Verification items for the finished model (mm, model axes). Face numbers are marked on the shaded views. A direction names the side the tool comes from. Round coordinates to 2 decimals unless told otherwise and drop trailing zeros. Order: outer loops, then holes, each group sorted by start corner. A loop starts at its lowest first (then second) coordinate and runs counter-clockwise, first axis right, second up. Notation, with made-up numbers: (-4, 18) -> (38, 18) arc R17 ccw to (38, 40) -> close; hole circle Ø5 at (6, 58). An arc over 180 degrees is marked (long way). Return JSON: item names as keys, results as strings. Group by question number.
Item 1: Sectioned sample at A-A on x = 0. Record the cut outline in (y, z).
Item 2: Depth check by flat-ended pin: pin 1 Ø1 at (x, z) = (-5, 0.5) entering from -Y. Enter the tip coordinate at first touch or a pass-through.
Item 3: Sectioned sample at C-C on z = 0.5. Record the cut outline in (x, y) (1 decimal), plus the area to 3 significant figures.
Item 4: Sectioned sample at B-B on y = 0. Record the cut outline in (x, z) (3 decimals), plus the area to 4 significant figures.
Item 5: Access from +Z, -Z, +X, -X, +Y, -Y to the whole of each face (thin tool, end or side, straight path). Record for the marked faces 1 and 2.
Item 6: Scan lines: probe 1 along Y at (x, z) = (4.5, 1); probe 2 along Y at (x, z) = (0.75, 1.05); probe 3 along X at (y, z) = (1, 0.35) (3 decimals). Record each from-to range of solid material in increasing order. Write a range as from..to.
Item 7: Sectioned sample at D-D on y = 38. Record the cut outline in (x, z).
Item 8: Draft check along Y on the marked faces 3, 4 and 5. Enter one of: pulls with the +Y half, pulls with the -Y half, needs draft (parallel to the pull), parting line crosses it, or undercut.
```python
from build123d import *

# Parameters (mm, degrees)
F0_R     = 5.4
F1_DEPTH = 1.5
F3_DEPTH = 1.5
F6_DEPTH = 1.5
F7_R     = 1


with BuildPart() as f1:
    # F0 (on Top) → F1 (new body, symmetric)
    with BuildSketch(Plane.XY):
        Circle(F0_R)
        with BuildLine():
            ThreePointArc((1.525, 2.1057955741), (2.3157072354, 1.1821590418), (2.6, 0))
            ThreePointArc((2.6, 0), (2.3157072354, -1.1821590418), (1.525, -2.1057955741))
            ThreePointArc((1.525, -2.1057955741), (0, -2.6), (-1.525, -2.1057955741))
            ThreePointArc((-1.525, -2.1057955741), (-2.6, 0), (-1.525, 2.1057955741))
            ThreePointArc((-1.525, 2.1057955741), (0, 2.6), (1.525, 2.1057955741))
        make_face(mode=Mode.SUBTRACT)
        with BuildLine():
            Line((-1.525, -2.1057955741), (-1.525, 2.1057955741))
            ThreePointArc((-1.525, 2.1057955741), (-2.6, 0), (-1.525, -2.1057955741))
        make_face()
        with BuildLine():
            ThreePointArc((1.525, -2.1057955741), (2.3157072354, -1.1821590418), (2.6, 0))
            ThreePointArc((2.6, 0), (2.3157072354, 1.1821590418), (1.525, 2.1057955741))
            Line((1.525, 2.1057955741), (1.525, -2.1057955741))
        make_face()
    extrude(amount=F1_DEPTH, both=True)

    # F2 (on face) → F3 (join, through all)
    with BuildSketch(Plane.XY.offset(1.5)):
        with BuildLine():
            Line((3.0470652436, 35), (0, 35))
            Line((0, 35), (-3.0470652436, 35))
            Line((-3.0470652436, 35), (-2, 5.0159744816))
            ThreePointArc((-2, 5.0159744816), (0, 5.4), (2, 5.0159744816))
            Line((2, 5.0159744816), (3.0470652436, 35))
        make_face()
    extrude(amount=-F3_DEPTH)

    # F4: F1 across face


with BuildPart() as f1_1:
    add(f1.part)
    add(f1.part.mirror(Plane(origin=(0, 21.1536915462, 0), x_dir=(1, 0, 0), z_dir=(0, 0, -1))))

    # F5 (on Top) → F6 (join, symmetric)
    with BuildSketch(Plane.XY):
        Polygon((0, 47.5), (-7.5, 35), (7.5, 35), align=None)
    extrude(amount=F6_DEPTH, both=True)

    # F7 (call 1 of 3: OpenCascade refuses the feature's edges together)
    f7_edges = [f1_1.edges().sort_by_distance(p)[0] for p in [
        (0, 47.5, 0),
    ]]
    fillet(f7_edges, radius=F7_R)

    # F7#2 (call 2 of 3)
    f7_2_edges = [f1_1.edges().sort_by_distance(p)[0] for p in [
        (7.5, 35, 0),
    ]]
    fillet(f7_2_edges, radius=F7_R)

    # F7#3 (call 3 of 3)
    f7_3_edges = [f1_1.edges().sort_by_distance(p)[0] for p in [
        (-5.273533, 35, -1.5),
    ]]
    fillet(f7_3_edges, radius=F7_R)


solid = f1_1.part
```
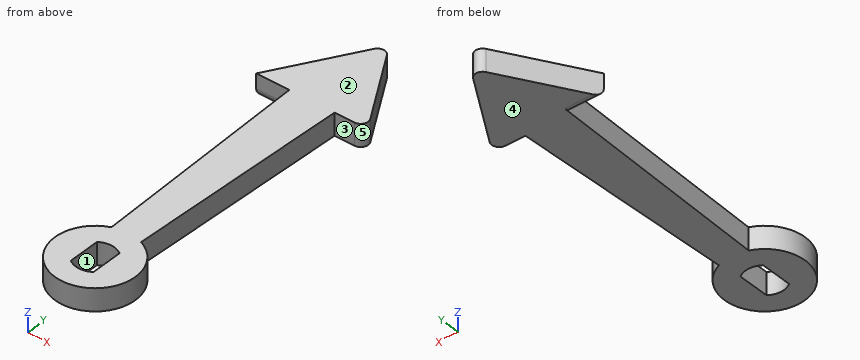
Recorded:
{
 "1": {"outline": "(-5.4, -1.5) -> (-2.6, -1.5) -> (-2.6, 1.5) -> (-5.4, 1.5) -> close; (2.6, -1.5) -> (46.56, -1.5) -> (46.56, 1.5) -> (2.6, 1.5) -> close"},
 "2": {"pin 1": "y = -2.98"},
 "3": {"outline": "(-7.5, 35) -> (-3, 35) -> (-2, 5) arc R5.4 ccw (long way) to (2, 5) -> (3, 35) -> (5.7, 35) arc R1 ccw to (6.6, 36.5) -> (0.9, 46.1) arc R1 ccw to (-0.9, 46.1) -> close; hole (-1.5, -2.1) arc R2.6 ccw to (1.5, -2.1) -> (1.5, 2.1) arc R2.6 ccw to (-1.5, 2.1) -> close", "area": "319 mm²"},
 "4": {"outline": "(-5.4, -1.5) -> (-1.525, -1.5) -> (-1.525, 1.5) -> (-5.4, 1.5) -> close; (1.525, -1.5) -> (5.4, -1.5) -> (5.4, 1.5) -> (1.525, 1.5) -> close", "area": "23.25 mm²"},
 "5": {"face 1": "+Z, -Z", "face 2": "+Z, +X, -X, +Y, -Y"},
 "6": {"probe 1": "-2.98..2.98, 35..40", "probe 2": "-5.35..-2.49, 2.49..46.22", "probe 3": "-5.307..-1.525, 1.525..5.307"},
 "7": {"outline": "(-5.7, -1.5) -> (5.7, -1.5) -> (5.7, 1.5) -> (-5.7, 1.5) -> close"},
 "8": {"face 3": "undercut", "face 4": "needs draft", "face 5": "parting line crosses it"}
}
